Could you check a few things on this model? Use its own coordinates, in mm. A direction names the side the tool comes from. Coordinates: 2 decimals unless noted, no trailing zeros. Order: outer loops, then holes, each group sorted by start corner. A loop starts at its lowest first (then second) coordinate and runs counter-clockwise, first axis right, second up. Notation, with made-up numbers: (-16.75, 29.25) -> (2.25, 29.25) arc R9 ccw to (2.25, 46.25) -> close; hole circle Ø8 at (60.25, 9). An arc over 180 degrees is marked (long way). Return JSON: item names as keys, results as strings. Group by question number.
from build123d import *

# Parameters (mm, degrees)
SKETCH1_W           = 40
SKETCH1_H           = 30
BOSS_EXTRUDE1_DEPTH = 6
SKETCH2_R           = 1.5
CUT_EXTRUDE1_DEPTH  = 6
FILLET1_R           = 4
SKETCH3_W           = 21
SKETCH3_H           = 21
CUT_EXTRUDE2_DEPTH  = 4
SKETCH4_W           = 7
SKETCH4_H           = 4.5
CUT_EXTRUDE3_DEPTH  = 2


with BuildPart() as part:
    # Sketch1 → Boss-Extrude1 (new body)
    with BuildSketch(Plane(origin=(0, 0, 0), x_dir=(1, 0, 0), z_dir=(0, 1, 0))):
        with Locations((20, 15)):
            Rectangle(SKETCH1_W, SKETCH1_H)
    extrude(amount=BOSS_EXTRUDE1_DEPTH)

    # Sketch2 → Cut-Extrude1 (cut)
    with BuildSketch(Plane(origin=(0, 6, 0), x_dir=(1, 0, 0), z_dir=(0, 1, 0))):
        with Locations(Location((5, 5, 0), (0, 0, 270))):
            Circle(SKETCH2_R)
        with Locations(Location((5, 25, 0), (0, 0, 90))):
            Circle(SKETCH2_R)
        with Locations(Location((35, 5, 0), (0, 0, 90))):
            Circle(SKETCH2_R)
        with Locations(Location((35, 25, 0), (0, 0, 270))):
            Circle(SKETCH2_R)
    extrude(amount=-CUT_EXTRUDE1_DEPTH, mode=Mode.SUBTRACT)

    # Fillet1
    fillet1_edges = [part.edges().sort_by_distance(p)[0] for p in [
        (0, 3, -30),
        (40, 3, -30),
        (40, 3, 0),
        (0, 3, 0),
    ]]
    fillet(fillet1_edges, radius=FILLET1_R)

    # Sketch3 → Cut-Extrude2 (cut)
    with BuildSketch(Plane(origin=(0, 6, 0), x_dir=(1, 0, 0), z_dir=(0, 1, 0))):
        with Locations((20, 15)):
            Rectangle(SKETCH3_W, SKETCH3_H)
    extrude(amount=-CUT_EXTRUDE2_DEPTH, mode=Mode.SUBTRACT)

    # Sketch4 → Cut-Extrude3 (cut)
    with BuildSketch(Plane(origin=(0, 6, 0), x_dir=(1, 0, 0), z_dir=(0, 1, 0))):
        with Locations((20, 2.25)):
            Rectangle(SKETCH4_W, SKETCH4_H)
    extrude(amount=-CUT_EXTRUDE3_DEPTH, mode=Mode.SUBTRACT)


solid = part.part
Q1. On a 3-axis mill with a long thin cutter (end or side, diameter ignored), from which of +Z, -Z, +X, -X, +Y, -Y can I reach the whole of each face in a straight line? I mean faces 5 (the flat face through (19.9, 3.6, -4.5)), 6 (the cylindrical face through (34.1, 3, -26.2)), 7 (the flat face through (16.5, 5, -2)). Say none if no direction works.
Q2. I want a section at B-B on y = 4.7. Please give me the cut outline in (x, z).
Q3. We'd pull the mould along Z, two halves only. Please class faces 1 (the cylindrical face through (38.797, 3.042, -28.859)), 2 (the flat face through (20, 2, -15)), 3 (the flat face through (23.5, 5, -2)), 4 (the cylindrical face through (4.93, 3.04, -23.5)): pulls with the +Z half, pulls with the -Z half, needs draft (parallel to the pull), parting line crosses it, or undercut.
Q4. I need wall thicknesses on line 1 along X through (y, z) = (3.95, -5); line 2 along Z through (x, y) = (4.5, 4.65); line 3 along X through (y, z) = (3.1, -9.25). Which ranges of each line are inside material? Lowest first, please. Write a range as from..to.
Q5. I'm going to push flat-ended pins straight in: pin 1 Ø1.6 at (y, z) = (5, -1.5) entering from +X; pin 2 Ø1.8 at (x, z) = (35, -25) entering from +Y; pin 3 Ø1.3 at (x, z) = (21.5, -3) entering from +Y; pin 4 Ø17 at (x, z) = (21.5, -14) entering from +Y. Where does each tip first touch, or does it pass through?
Q6. I want a section at C-C on z = -5. Please give me the cut outline in (x, y), and give its area (3 significant figures).
Q7. I want a section at D-D on y = 2.75. Please give me the cut outline in (x, z), and give its area (3 significant figures).
Q8. I want a section at A-A on x = 35. Please give me the cut outline in (y, z), and give its area (3 significant figures).
Response values:
{
 "1": {"face 5": "+Y", "face 6": "+Y, -Y", "face 7": "+Z, +Y"},
 "2": {"outline": "(0, -26) arc R4 ccw to (4, -30) -> (36, -30) arc R4 ccw to (40, -26) -> (40, -4) arc R4 ccw to (36, 0) -> (23.5, 0) -> (23.5, -4.5) -> (30.5, -4.5) -> (30.5, -25.5) -> (9.5, -25.5) -> (9.5, -4.5) -> (16.5, -4.5) -> (16.5, 0) -> (4, 0) arc R4 ccw to (0, -4) -> close; hole circle Ø3 at (5, -25); hole circle Ø3 at (5, -5); hole circle Ø3 at (35, -25); hole circle Ø3 at (35, -5)"},
 "3": {"face 1": "pulls with the -Z half", "face 2": "undercut", "face 3": "needs draft", "face 4": "undercut"},
 "4": {"line 1": "x = 0..3.5, 6.5..9.5, 30.5..33.5, 36.5..40", "line 2": "z = -30..-26.41, -23.59..-6.41, -3.59..0", "line 3": "x = 0..9.5, 30.5..40"},
 "5": {"pin 1": "stops at x = 39.62", "pin 2": "passes through", "pin 3": "stops at y = 4", "pin 4": "stops at y = 2"},
 "6": {"outline": "(0, 0) -> (3.5, 0) -> (3.5, 6) -> (0, 6) -> close; (6.5, 0) -> (33.5, 0) -> (33.5, 6) -> (30.5, 6) -> (30.5, 2) -> (9.5, 2) -> (9.5, 6) -> (6.5, 6) -> close; (36.5, 0) -> (40, 0) -> (40, 6) -> (36.5, 6) -> close", "area": "120 mm²"},
 "7": {"outline": "(0, -26) arc R4 ccw to (4, -30) -> (36, -30) arc R4 ccw to (40, -26) -> (40, -4) arc R4 ccw to (36, 0) -> (4, 0) arc R4 ccw to (0, -4) -> close; hole circle Ø3 at (5, -25); hole circle Ø3 at (5, -5); hole (9.5, -25.5) -> (30.5, -25.5) -> (30.5, -4.5) -> (9.5, -4.5) -> close; hole circle Ø3 at (35, -25); hole circle Ø3 at (35, -5)", "area": "717 mm²"},
 "8": {"outline": "(0, -30) -> (6, -30) -> (6, -26.5) -> (0, -26.5) -> close; (0, -23.5) -> (6, -23.5) -> (6, -6.5) -> (0, -6.5) -> close; (0, -3.5) -> (6, -3.5) -> (6, 0) -> (0, 0) -> close", "area": "144 mm²"}
}
